Part print with two shaded views. Sizes in mm from the minimum x, y, z corner. Round coordinates to 2 decimals unless told otherwise and drop trailing zeros. Order: outer loops, then holes, each group sorted by start corner. A loop starts at its lowest first (then second) coordinate and runs counter-clockwise, first axis right, second up. Notation, with made-up numbers: (-1, -10) -> (29, -10) arc R20 cw to (29, 13) -> close; hole circle Ø10 at (20.5, -12.75). An arc over 180 degrees is marked (long way). Use a Markdown table: item, result. Add a question column.
Item 1: Slice it at C-C, the plane y = 1.5. Give the cut face in (x, z).
Item 2: Slice it at D-D, the plane x = 1.65. Give the cut face in (y, z), plus the area to 3 significant figures.
Item 3: Slice it at B-B, the plane z = 7.25. Give the cut face in (x, y).
Item 4: Two-plate mould, pull along Y, no slides. Class the marked faces 1, 2, 3 and 4: released by +Y, released by -Y, zero draft, split by the parting line, or undercut.
Item 5: Slice it at A-A, the plane x = 3. Give the cut face in (y, z).
Item 6: Probe L1, parallel to Y at x = 3, z = 2; L2, parallel to X at y = 3, z = 6.25; L3, parallel to Y at x = 2.25, z = 1.5. List the from-to ranges inside material, lowest first.
Item 7: Pin check, flat tip, straight feed: pin 1 (1.5 mm diameter, centred on x = 1.5, z = 7, fed in from +Y). Stop position of the tip, or through.
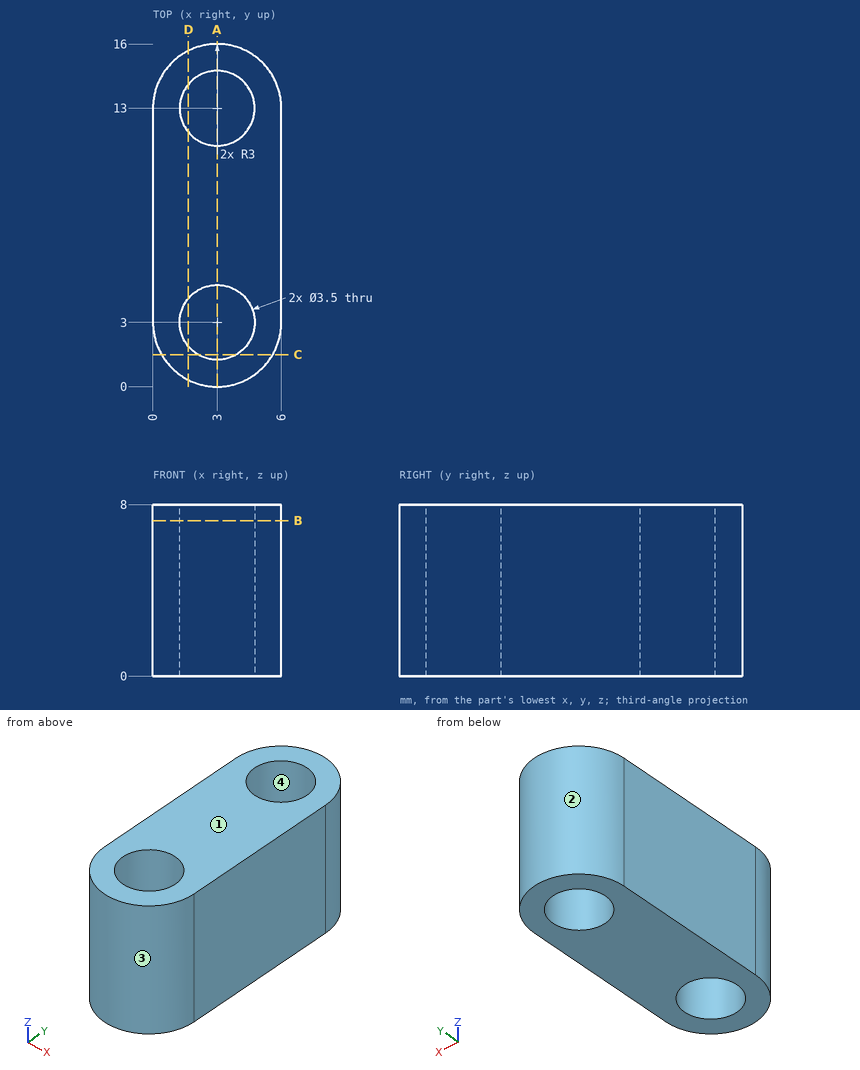
Check sheet entries:
| question | item | result |
|---|---|---|
| 1 | outline | (0.4, 0) -> (2.1, 0) -> (2.1, 8) -> (0.4, 8) -> close; (3.9, 0) -> (5.6, 0) -> (5.6, 8) -> (3.9, 8) -> close |
| 2 | outline | (0.32, 0) -> (1.89, 0) -> (1.89, 8) -> (0.32, 8) -> close; (4.11, 0) -> (11.89, 0) -> (11.89, 8) -> (4.11, 8) -> close; (14.11, 0) -> (15.68, 0) -> (15.68, 8) -> (14.11, 8) -> close |
| 2 | area | 87.2 mm2 |
| 3 | outline | (0, 3) arc R3 ccw to (6, 3) -> (6, 13) arc R3 ccw to (0, 13) -> close; hole circle Ø3.5 at (3, 3); hole circle Ø3.5 at (3, 13) |
| 4 | face 1 | zero draft |
| 4 | face 2 | released by +Y |
| 4 | face 3 | released by -Y |
| 4 | face 4 | undercut |
| 5 | outline | (0, 0) -> (1.25, 0) -> (1.25, 8) -> (0, 8) -> close; (4.75, 0) -> (11.25, 0) -> (11.25, 8) -> (4.75, 8) -> close; (14.75, 0) -> (16, 0) -> (16, 8) -> (14.75, 8) -> close |
| 6 | L1 | 0 to 1.25, 4.75 to 11.25, 14.75 to 16 |
| 6 | L2 | 0 to 1.25, 4.75 to 6 |
| 6 | L3 | 0.1 to 1.42, 4.58 to 11.42, 14.58 to 15.9 |
| 7 | pin 1 | y = 15.9 |
